Can you work these out from the drawing? Everything is in mm from the part's minimum corner. Give positions to 0.01 mm unless a question says otherwise; leave off trailing zeros. Write each loop counter-clockwise with the first axis right and the second up, starting at its lowest first coordinate (ties: lowest second). Pieces come first, ordered by that corner, then holes. Notation, with made-up numbers: (21.5, 87) -> (45.5, 87) arc R9 ccw to (45.5, 99) -> close; hole circle Ø1 at (-17.5, -6.5). An arc over 180 degrees is marked (long way). Use one line per item in the form item = value.
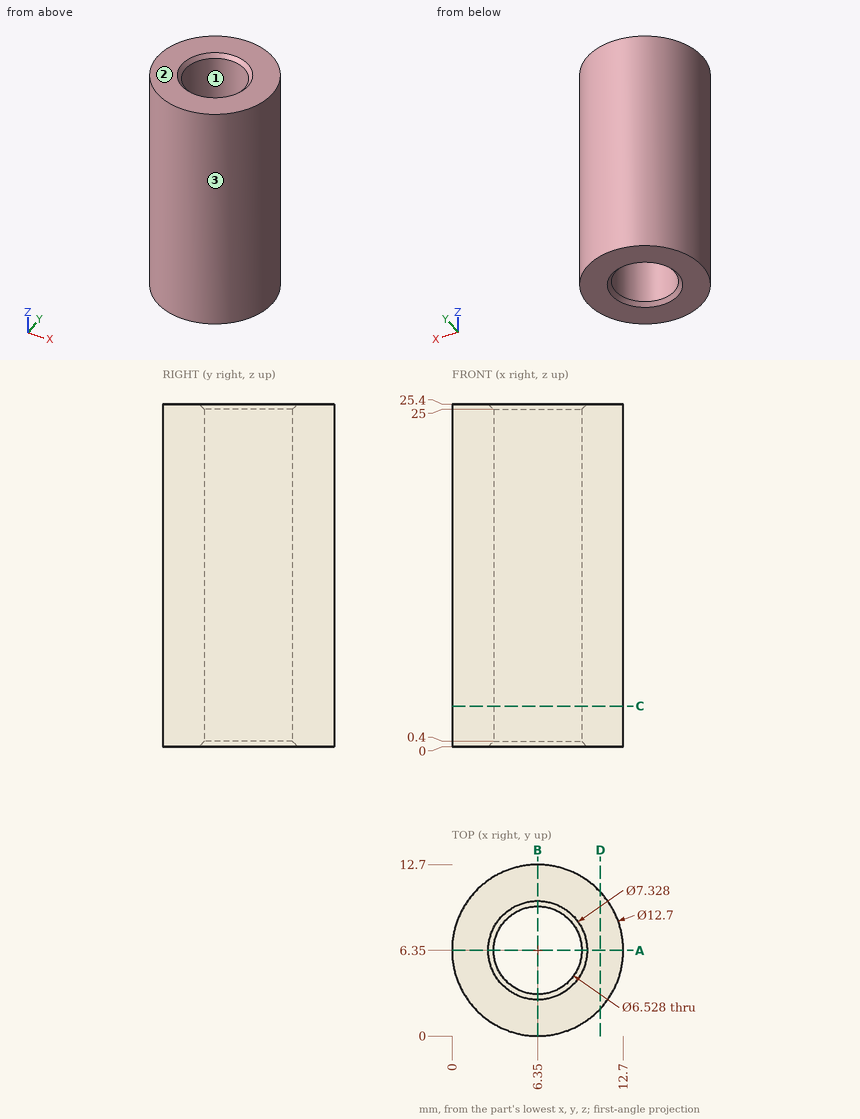
Q1. I want a section at A-A, the plane y = 6.35. Write out the boundary of the cut face in (x, z), and give its area (3 significant figures).
Result set:
outline = (0, 0) -> (2.69, 0) -> (3.09, 0.4) -> (3.09, 25) -> (2.69, 25.4) -> (0, 25.4) -> close; (9.61, 0.4) -> (10.01, 0) -> (12.7, 0) -> (12.7, 25.4) -> (10.01, 25.4) -> (9.61, 25) -> close
area = 156 mm2
Q2. Will these pins go through, and if not, where does the flat tip stop? pin 1 Ø3 at (y, z) = (8, 15.5) entering from +X; pin 2 Ø2 at (x, z) = (4, 10.5) entering from +Y (1 decimal); pin 3 Ø1 at (x, z) = (9, 14) entering from -Y (3 decimals).
Result set:
pin_1 = 12.7
pin_2 = 12.6
pin_3 = 0.375
Q3. If we mould it in two halves opening along X, with no side actions, what happens to the marked faces 1, 2 and 3? For each: +X half, -X half, draft (parallel to the pull), parting line (faces both ways), or undercut.
Result set:
face_1 = undercut
face_2 = draft
face_3 = parting line
Q4. I want a section at D-D, the plane x = 11. Write out the boundary of the cut face in (y, z), and give its area (3 significant figures).
Result set:
outline = (2.03, 0) -> (10.67, 0) -> (10.67, 25.4) -> (2.03, 25.4) -> close
area = 220 mm2
Q5. I want a section at C-C, the plane z = 3. Write out the boundary of the cut face in (x, y).
Result set:
outline = circle Ø12.7 at (6.35, 6.35); hole circle Ø6.53 at (6.35, 6.35)
Q6. If I drill on line 1 along Y through (x, z) = (6.35, 19.5); line 2 along Y through (x, z) = (8.75, 22.75), over which ranges is the centre line in solid material (lowest first)? Write a range as from..to.
Result set:
line_1 = 0..3.09, 9.61..12.7
line_2 = 0.47..4.14, 8.56..12.23
